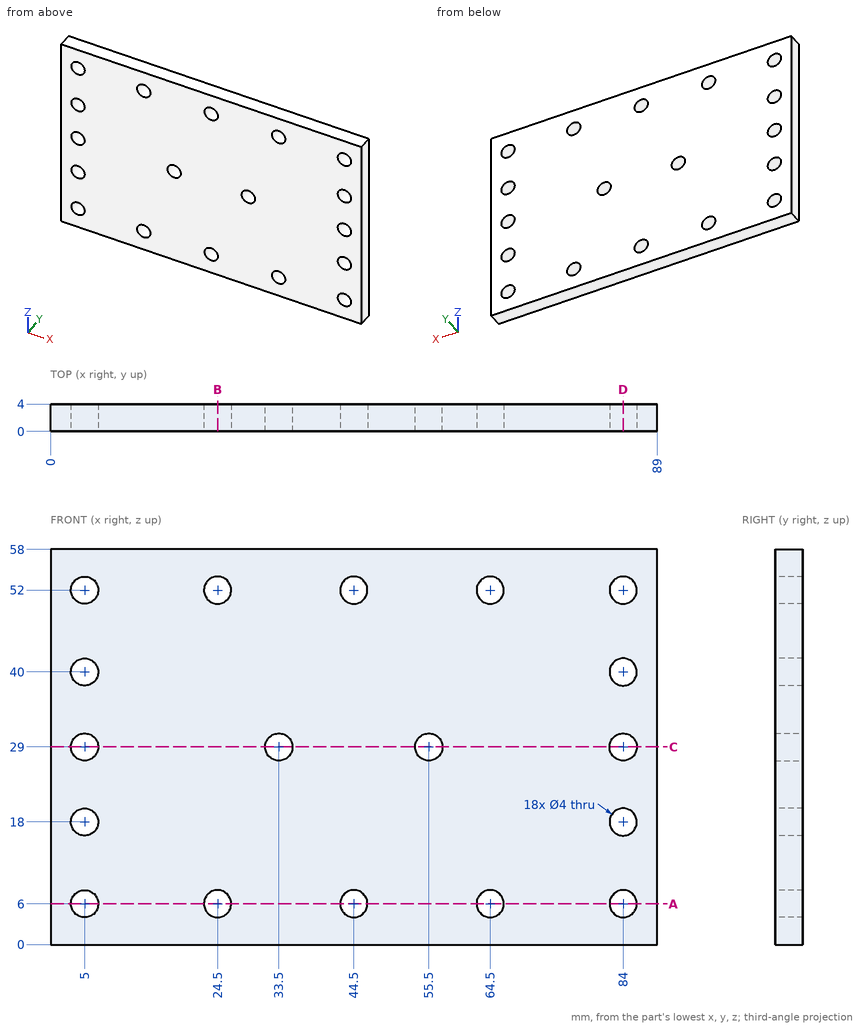
Check sheet for the drawn part. Datum: minimum x, y, z corner. Units: mm. Round coordinates to 2 decimals unless told otherwise and drop trailing zeros. Write each loop counter-clockwise with the first axis right and the second up, starting at its lowest first coordinate (ties: lowest second). Pieces come first, ordered by that corner, then holes. Notation, with made-up numbers: (14.5, 26.5) -> (31.5, 26.5) arc R27 cw to (31.5, 62.5) -> close; hole circle Ø11 at (-38.5, 22.5). An arc over 180 degrees is marked (long way). One line per item, written item: value. Start each with the question number.
(1) Scan lines: line 1 (Z direction, x = 24.5, y = 0.85); line 2 (X direction, y = 2.2, z = 6); line 3 (X direction, y = 2.5, z = 29). Record each from-to range of solid material in increasing order. Write a range as [from, to].
(2) Cross-section at A-A, the plane z = 6. Record the cut outline in (x, y).
(3) Cross-section at D-D, the plane x = 84. Record the cut outline in (y, z), and give its area (3 significant figures).
(4) Cross-section at C-C, the plane z = 29. Record the cut outline in (x, y), and give its area (3 significant figures).
(5) Cross-section at B-B, the plane x = 24.5. Record the cut outline in (y, z).
Answer:
1. line 1: [0, 4], [8, 50], [54, 58]
1. line 2: [0, 3], [7, 22.5], [26.5, 42.5], [46.5, 62.5], [66.5, 82], [86, 89]
1. line 3: [0, 3], [7, 31.5], [35.5, 53.5], [57.5, 82], [86, 89]
2. outline: (0, 0) -> (3, 0) -> (3, 4) -> (0, 4) -> close; (7, 0) -> (22.5, 0) -> (22.5, 4) -> (7, 4) -> close; (26.5, 0) -> (42.5, 0) -> (42.5, 4) -> (26.5, 4) -> close; (46.5, 0) -> (62.5, 0) -> (62.5, 4) -> (46.5, 4) -> close; (66.5, 0) -> (82, 0) -> (82, 4) -> (66.5, 4) -> close; (86, 0) -> (89, 0) -> (89, 4) -> (86, 4) -> close
3. outline: (0, 0) -> (4, 0) -> (4, 4) -> (0, 4) -> close; (0, 8) -> (4, 8) -> (4, 16) -> (0, 16) -> close; (0, 20) -> (4, 20) -> (4, 27) -> (0, 27) -> close; (0, 31) -> (4, 31) -> (4, 38) -> (0, 38) -> close; (0, 42) -> (4, 42) -> (4, 50) -> (0, 50) -> close; (0, 54) -> (4, 54) -> (4, 58) -> (0, 58) -> close
3. area: 152 mm²
4. outline: (0, 0) -> (3, 0) -> (3, 4) -> (0, 4) -> close; (7, 0) -> (31.5, 0) -> (31.5, 4) -> (7, 4) -> close; (35.5, 0) -> (53.5, 0) -> (53.5, 4) -> (35.5, 4) -> close; (57.5, 0) -> (82, 0) -> (82, 4) -> (57.5, 4) -> close; (86, 0) -> (89, 0) -> (89, 4) -> (86, 4) -> close
4. area: 292 mm²
5. outline: (0, 0) -> (4, 0) -> (4, 4) -> (0, 4) -> close; (0, 8) -> (4, 8) -> (4, 50) -> (0, 50) -> close; (0, 54) -> (4, 54) -> (4, 58) -> (0, 58) -> close
